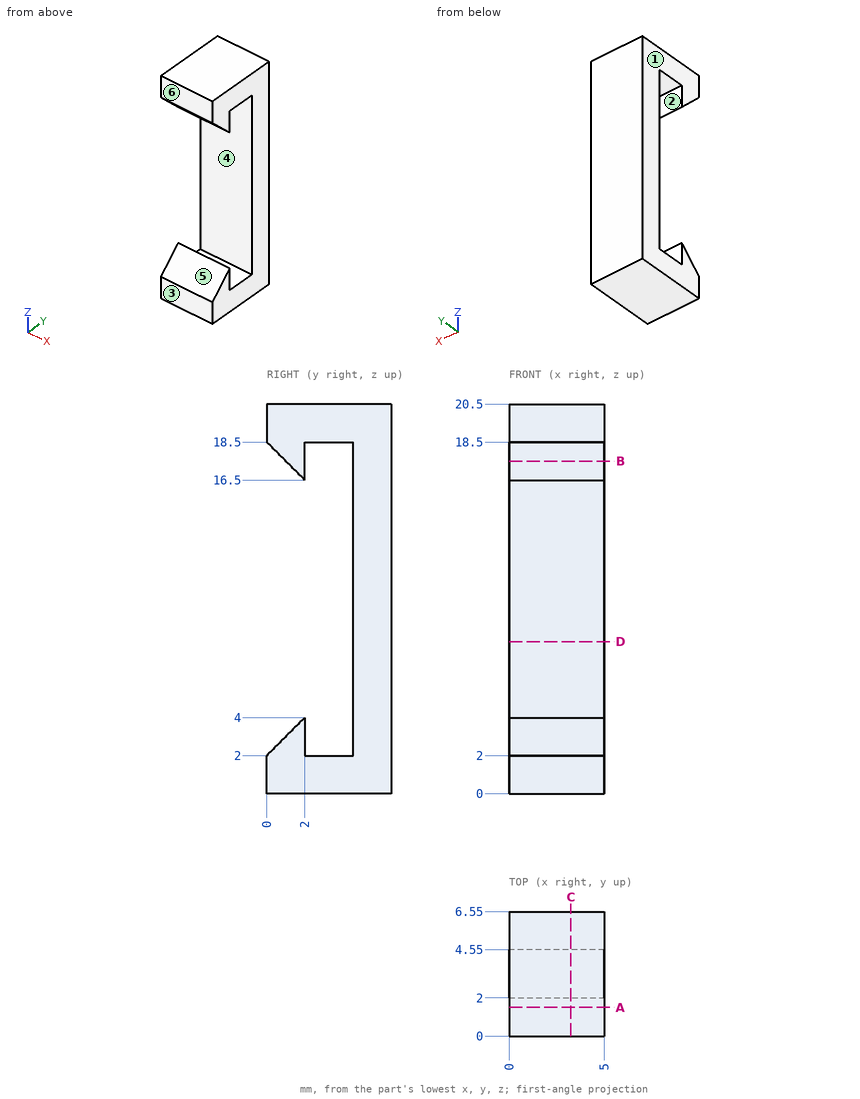
Design review of the part shown in the three views and the two pictorial views. Dimensions are in mm from the part's minimum x, y and z. A direction names the side the tool comes from. Give positions to 0.01 mm unless a question says otherwise; leave off trailing zeros. Loops run counter-clockwise (first coordinate to the right, second up) from the corner with the lowest first, then second, coordinate; pieces in that order, holes last. Notation, with made-up numbers: M 72.25,-27.5 L 127.25,-27.5 A20 ccw 127.25,-22.5 Z; hole C 24,12 d9. An arc over 180 degrees is marked long. Put each result on its own line as item: value. Start each with the question number.
(1) Add section A-A, the plane y = 1.5. Write out the cut boundary in (x, z), then the cut area to 3 significant figures.
(2) The part is to be moulded in two halves that separate along Y. For the marked faces 1, 2 and 3, say which applies: +Y half, -Y half, draft (parallel to the pull), parting line (faces both ways), or undercut.
(3) Wall thickness on L1, parallel to Z at x = 2.85, y = 4; L2, parallel to Y at x = 3.75, z = 9.5; L3, parallel to Z at x = 1.8, y = 1: over which ranges is each line inside the solid? List them lowest first.
(4) Add section C-C, the plane x = 3.25. Write out the cut boundary in (y, z), then the cut area to 3 significant figures.
(5) Add section D-D, the plane z = 8. Write out the cut boundary in (x, y), then the cut area to 3 significant figures.
(6) Machinability: for the marked faces 4, 5 and 6, which of the approach directions +Z, -Z, +X, -X, +Y, -Y give a long, thin tool a straight path to every point of the face, cutting with its end or side? Answer none if there is none.
(7) For pin 1 (2.5 mm diameter, centred on x = 2.5, z = 13, fed in from -Y), flat-tipped, find the tip position at first contact; note if it passes through.
(8) Add section B-B, the plane z = 17.5. Write out the cut boundary in (x, y), then the cut area to 3 significant figures.
Result:
1. outline: M 0,0 L 5,0 L 5,3.5 L 0,3.5 Z; M 0,17 L 5,17 L 5,20.5 L 0,20.5 Z
1. area: 35.0 mm^2
2. face 1: draft
2. face 2: undercut
2. face 3: -Y half
3. L1: z = 0 to 2, 18.5 to 20.5
3. L2: y = 4.55 to 6.55
3. L3: z = 0 to 3, 17.5 to 20.5
4. outline: M 0,0 L 6.55,0 L 6.55,20.5 L 0,20.5 L 0,18.5 L 2,16.5 L 2,18.5 L 4.55,18.5 L 4.55,2 L 2,2 L 2,4 L 0,2 Z
4. area: 63.2 mm^2
5. outline: M 0,4.55 L 5,4.55 L 5,6.55 L 0,6.55 Z
5. area: 10.0 mm^2
6. face 4: +X, -X
6. face 5: +X, -X, -Y
6. face 6: +Z, -Z, +X, -X, -Y
7. pin 1: stops at y = 4.55
8. outline: M 0,1 L 5,1 L 5,2 L 0,2 Z; M 0,4.55 L 5,4.55 L 5,6.55 L 0,6.55 Z
8. area: 15.0 mm^2
